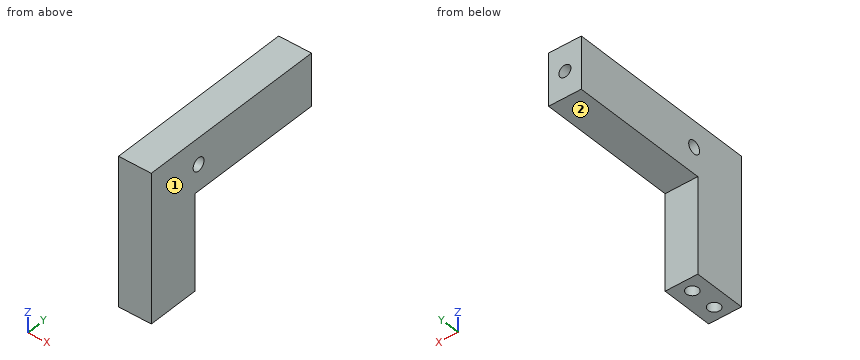
from build123d import *

# Parameters (mm, degrees)
SKETCH1_W                       = 9.525
SKETCH1_H                       = 15.24
EXTRUDE1_DEPTH                  = 43.18
SKETCH4_W                       = 9.525
SKETCH4_H                       = 15.24
EXTRUDE2_DEPTH                  = 40.64
F_6_32_TAPPED_HOLE1_D           = 2.7051
F_6_32_TAPPED_HOLE1_DEPTH       = 13.97
F_6_32_TAPPED_HOLE1_CBORE_D     = 3.5052
F_6_32_TAPPED_HOLE1_CBORE_DEPTH = 9.906
F_6_32_TAPPED_HOLE1_TIP         = 0.81269403
F_6_CLEARANCE_HOLE1_D           = 3.7973
F_6_CLEARANCE_HOLE1_DEPTH       = 9.906
F_6_CLEARANCE_HOLE1_TIP         = 1.140824014
F_6_32_TAPPED_HOLE2_D           = 2.7051
F_6_32_TAPPED_HOLE2_DEPTH       = 13.97
F_6_32_TAPPED_HOLE2_CBORE_D     = 3.5052
F_6_32_TAPPED_HOLE2_CBORE_DEPTH = 9.906
F_6_32_TAPPED_HOLE2_TIP         = 0.81269403


with BuildPart() as part:
    # Sketch1 → Extrude1 (new body)
    with BuildSketch(Plane.XY):
        with Locations((-4.7625, 7.62)):
            Rectangle(SKETCH1_W, SKETCH1_H)
    extrude(amount=EXTRUDE1_DEPTH)

    # Sketch4 → Extrude2 (add)
    with BuildSketch(Plane(origin=(0, 15.24, 0), x_dir=(-1, 0, 0), z_dir=(0, 1, 0))):
        with Locations((4.7625, 35.56)):
            Rectangle(SKETCH4_W, SKETCH4_H)
    extrude(amount=EXTRUDE2_DEPTH)

    # #6-32 Tapped Hole1
    with Locations(Plane(origin=(-4.7625, 11.43, 0), x_dir=(-1, 0, 0), z_dir=(0, 0, -1))):
        with Locations((0, 0), (0, -7.62), (15.003961831, 4.683879058)):
            CounterBoreHole(F_6_32_TAPPED_HOLE1_D / 2, F_6_32_TAPPED_HOLE1_CBORE_D / 2, F_6_32_TAPPED_HOLE1_CBORE_DEPTH, depth=F_6_32_TAPPED_HOLE1_DEPTH)
            with Locations((0, 0, -(F_6_32_TAPPED_HOLE1_DEPTH + F_6_32_TAPPED_HOLE1_TIP / 2))):  # 118° drill point
                Cone(0, F_6_32_TAPPED_HOLE1_D / 2, F_6_32_TAPPED_HOLE1_TIP, mode=Mode.SUBTRACT)

    # #6 Clearance Hole1
    with Locations(Plane(origin=(0, 16.51, 35.56), x_dir=(0, 1, 0), z_dir=(1, 0, 0))):
        with Locations((0, 0)):
            Hole(F_6_CLEARANCE_HOLE1_D / 2, depth=F_6_CLEARANCE_HOLE1_DEPTH)
            with Locations((0, 0, -(F_6_CLEARANCE_HOLE1_DEPTH + F_6_CLEARANCE_HOLE1_TIP / 2))):  # 118° drill point
                Cone(0, F_6_CLEARANCE_HOLE1_D / 2, F_6_CLEARANCE_HOLE1_TIP, mode=Mode.SUBTRACT)

    # #6-32 Tapped Hole2
    with Locations(Plane(origin=(-4.7625, 55.88, 35.56), x_dir=(1, 0, 0), z_dir=(0, 1, 0))):
        with Locations((0, 0)):
            CounterBoreHole(F_6_32_TAPPED_HOLE2_D / 2, F_6_32_TAPPED_HOLE2_CBORE_D / 2, F_6_32_TAPPED_HOLE2_CBORE_DEPTH, depth=F_6_32_TAPPED_HOLE2_DEPTH)
            with Locations((0, 0, -(F_6_32_TAPPED_HOLE2_DEPTH + F_6_32_TAPPED_HOLE2_TIP / 2))):  # 118° drill point
                Cone(0, F_6_32_TAPPED_HOLE2_D / 2, F_6_32_TAPPED_HOLE2_TIP, mode=Mode.SUBTRACT)


solid = part.part
The model under review builds one solid part; all positions refer to its coordinate system, in mm. Face numbers are marked on the shaded views. A direction names the side the tool comes from. Round coordinates to 2 decimals unless told otherwise and drop trailing zeros. Loops run counter-clockwise (first coordinate to the right, second up) from the corner with the lowest first, then second, coordinate; pieces in that order, holes last. Notation, with made-up numbers: (78, 18.5) -> (110, 18.5) arc R15 ccw to (110, 32.5) -> close; hole circle Ø2 at (33, -26.75). An arc over 180 degrees is marked (long way). One line per question, with ' | ' between items. Start each with the question number.
Item 1: For pin 1 (2 mm diameter, centred on x = -4, y = 34.5, fed in from -Z); pin 2 (1.1 mm diameter, centred on x = -5, y = 12, fed in from -Z); pin 3 (3 mm diameter, centred on x = -4.76, y = 3.81, fed in from -Z), all flat-tipped, find the tip position at first contact; note any pin that passes through.
Item 2: Machinability: for the marked faces 1 and 2, which of the approach directions +Z, -Z, +X, -X, +Y, -Y give a long, thin tool a straight path to every point of the face, cutting with its end or side? Answer none if there is none.
Item 3: Add section B-B, the plane z = 11.5. Write out the cut boundary in (x, y) (1 decimal), then the cut area to 3 significant figures.
Item 4: Wall thickness on line 1 along Z through (x, y) = (-5, 16.51); line 2 along X through (y, z) = (44.55, 35.56) (3 decimals); line 3 along X through (y, z) = (52, 35.56) (3 decimals): over which ranges is each line inside the solid? List them lowest first. Write a range as [from, to].
Item 5: Add section C-C, the plane y = 32. Write out the cut boundary in (x, z) (3 decimals), then the cut area to 3 significant figures.
Item 6: Add section A-A, the plane y = 50. Write out the cut boundary in (x, z) (1 decimal).
Item 7: Add section D-D, the plane z = 20. Write out the cut boundary in (x, y) (3 decimals), then the cut area to 3 significant figures.
Return value:
1) pin 1: stops at z = 27.94 | pin 2: stops at z = 14.08 | pin 3: stops at z = 9.91
2) face 1: +Z, -Z, +X, +Y, -Y | face 2: -Z, +X, -X, +Y
3) outline: (-9.5, 0) -> (0, 0) -> (0, 15.2) -> (-9.5, 15.2) -> close; hole circle Ø2.7 at (-4.8, 3.8); hole circle Ø2.7 at (-4.8, 11.4) | area: 134 mm2
4) line 1: z = [27.94, 33.66], [37.46, 43.18] | line 2: x = [-9.525, -6.115], [-3.41, 0] | line 3: x = [-9.525, -6.515], [-3.01, 0]
5) outline: (-9.525, 27.94) -> (0, 27.94) -> (0, 43.18) -> (-9.525, 43.18) -> close | area: 145 mm2
6) outline: (-9.5, 27.9) -> (0, 27.9) -> (0, 43.2) -> (-9.5, 43.2) -> close; hole circle Ø3.5 at (-4.8, 35.6)
7) outline: (-9.525, 0) -> (0, 0) -> (0, 15.24) -> (-9.525, 15.24) -> close | area: 145 mm2
